```python
from build123d import *

# Parameters (mm, degrees)
CROQUIS1_R               = 1.598160281
CROQUIS1_R_2             = 1.600993429
CROQUIS1_R_3             = 1.650918845
SALIENTE_EXTRUIR7_DEPTH  = 2
CROQUIS2_R               = 5.764999893
CROQUIS2_R_2             = 1.651186543
SALIENTE_EXTRUIR8_DEPTH  = 7.7
SALIENTE_EXTRUIR9_DEPTH  = 26.3
CROQUIS6_R               = 0.999415005
SALIENTE_EXTRUIR10_DEPTH = 6.4


with BuildPart() as part:
    # Croquis1 → Saliente-Extruir7 (new body)
    with BuildSketch(Plane.XY):
        with BuildLine():
            Line((4.00000019, 5.763000809), (10.195969576, 3.8191034))
            ThreePointArc((10.195969576, 3.8191034), (12.999977706, 0.001566069), (10.197782, -3.817301838))
            Line((10.197782, -3.817301838), (4.00000019, -5.764999893))
            Line((4.00000019, -5.764999893), (-4.00000019, -5.764999893))
            Line((-4.00000019, -5.764999893), (-10.199065979, -3.817665654))
            ThreePointArc((-10.199065979, -3.817665654), (-13.000622723, -0.001109837), (-10.199143851, 3.815503142))
            Line((-10.199143851, 3.815503142), (-4.00000019, 5.763000809))
            Line((-4.00000019, 5.763000809), (4.00000019, 5.763000809))
        make_face()
        with Locations((8.997973452, 0.000616233)):
            Circle(CROQUIS1_R, mode=Mode.SUBTRACT)
        with Locations((-9.000145119, -0.001069025)):
            Circle(CROQUIS1_R_2, mode=Mode.SUBTRACT)
        Circle(CROQUIS1_R_3, mode=Mode.SUBTRACT)
    extrude(amount=-SALIENTE_EXTRUIR7_DEPTH)

    # Croquis2 → Saliente-Extruir8 (add)
    with BuildSketch(Plane(origin=(0, 0, -2), x_dir=(-1, 0, 0), z_dir=(0, 0, -1))):
        with Locations(Location((0, 0, 0), (0, 0, 91.508919394))):
            Circle(CROQUIS2_R)
        with Locations(Location((0, 0, 0), (0, 0, 180))):
            Circle(CROQUIS2_R_2, mode=Mode.SUBTRACT)
    extrude(amount=SALIENTE_EXTRUIR8_DEPTH)

    # Croquis3 → Saliente-Extruir9 (add)
    with BuildSketch(Plane(origin=(0, 0, -9.7), x_dir=(-1, 0, 0), z_dir=(0, 0, -1))):
        with BuildLine():
            Line((3.526868458, 5.783774708), (-3.526868458, 5.783774708))
            ThreePointArc((-3.526868458, 5.783774708), (-5.648188802, 4.905095052), (-6.526868458, 2.783774708))
            Line((-6.526868458, 2.783774708), (-6.526868458, -4.783774708))
            ThreePointArc((-6.526868458, -4.783774708), (-6.233975239, -5.490881489), (-5.526868458, -5.783774708))
            Line((-5.526868458, -5.783774708), (5.526868458, -5.783774708))
            ThreePointArc((5.526868458, -5.783774708), (6.233975239, -5.490881489), (6.526868458, -4.783774708))
            Line((6.526868458, -4.783774708), (6.526868458, 2.783774708))
            ThreePointArc((6.526868458, 2.783774708), (5.648188802, 4.905095052), (3.526868458, 5.783774708))
        make_face()
    extrude(amount=SALIENTE_EXTRUIR9_DEPTH)

    # Croquis5 → Cortar-Revolución1 (revolve, cut)
    with BuildSketch(Plane(origin=(0, 0, 0), x_dir=(1, 0, 0), z_dir=(0, 1, 0)), mode=Mode.PRIVATE) as cortar_revoluci_n1_sk:
        Polygon((-3.5, 36), (-8.472559386, 30.803521887), (-8.472559386, 36), align=None)
    revolve(cortar_revoluci_n1_sk.sketch.rotate(Axis((0, 0, -39.9199001), (0, 0, 1)), 203.098732746), axis=Axis((0, 0, -39.9199001), (0, 0, 1)), mode=Mode.SUBTRACT)

    # Croquis6 → Saliente-Extruir10 (add)
    with BuildSketch(Plane(origin=(0, 0, -36), x_dir=(-1, 0, 0), z_dir=(0, 0, -1))):
        Circle(CROQUIS6_R)
    extrude(amount=SALIENTE_EXTRUIR10_DEPTH)


solid = part.part
```
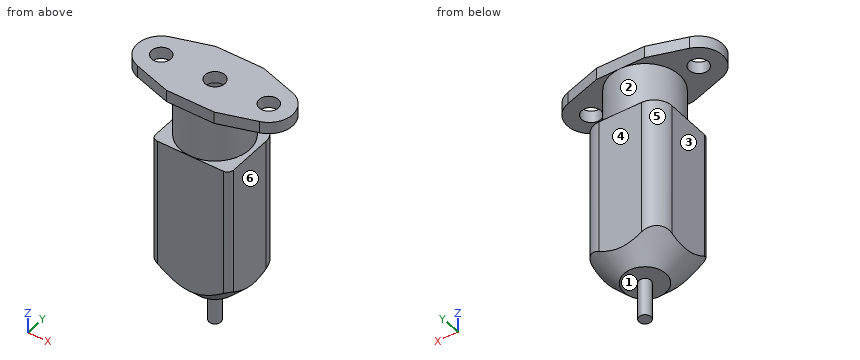
Model file for the job. Use its own axes, mm. Face numbers are marked on the shaded views. A direction names the side the tool comes from. Give positions to 0.01 mm unless a question says otherwise; leave off trailing zeros. Order: outer loops, then holes, each group sorted by start corner. A loop starts at its lowest first (then second) coordinate and runs counter-clockwise, first axis right, second up.
1) Pin check, flat tips, straight feed: pin 1 (6 mm diameter, centred on x = 4.5, y = 1.5, fed in from -Z); pin 2 (6 mm diameter, centred on y = -0.5, z = -20.5, fed in from -X); pin 3 (1 mm diameter, centred on x = 0, z = -0.5, fed in from -Y) (3 decimals). Stop position of each tip, or through.
2) 3-axis set-ups, long thin cutter, end or side, ignore diameter. For the marked faces 4, 5 and 6: which of +Z, -Z, +X, -X, +Y, -Y reach the whole face in a straight line?
3) Wall check: probe 1 along Y at (x, z) = (0, -0.5) (3 decimals); probe 2 along X at (y, z) = (-1.5, -11.5); probe 3 along X at (y, z) = (1.5, -5.5). Give the ranges that are in metal, low to high.
4) Mould opens along Z. For the marked faces 1, 2 and 3 say: +Z half, -Z half, draft (parallel to the pull), parting line (faces both ways), or undercut.
5) Saw through at A-A, the plane z = -12.5. Write the cut outline in (x, y), then the cut area to 3 significant figures.
Computed:
1. pin 1: stops at z = -36
1. pin 2: stops at x = -6.53
1. pin 3: stops at y = -5.765
2. face 4: +Z, -Z, +X, -X, +Y
2. face 5: -Z, -X, +Y
2. face 6: -Z, +X, +Y, -Y
3. probe 1: y = -5.765 to -1.651, 1.651 to 5.763
3. probe 2: x = -6.53 to 6.53
3. probe 3: x = -5.57 to -0.69, 0.69 to 5.57
4. face 1: -Z half
4. face 2: undercut
4. face 3: draft
5. outline: (-6.53, -4.78) arc R1 ccw to (-5.53, -5.78) - (5.53, -5.78) arc R1 ccw to (6.53, -4.78) - (6.53, 2.78) arc R3 ccw to (3.53, 5.78) - (-3.53, 5.78) arc R3 ccw to (-6.53, 2.78) - close
5. area: 147 mm2
